from build123d import *

# Parameters (mm, degrees)
F0_R     = 25
F1_DEPTH = 43.4


with BuildPart() as f1:
    # F0 (on Front) → F1 (new body)
    with BuildSketch(Plane.XZ):
        Circle(F0_R)
        with BuildLine():
            ThreePointArc((-11.4564392374, 5), (0, 12.5), (11.4564392374, 5))
            Line((11.4564392374, 5), (15, 5))
            Line((15, 5), (15, -5))
            Line((15, -5), (11.4564392374, -5))
            ThreePointArc((11.4564392374, -5), (0, -12.5), (-11.4564392374, -5))
            Line((-11.4564392374, -5), (-15, -5))
            Line((-15, -5), (-15, 5))
            Line((-15, 5), (-11.4564392374, 5))
        make_face(mode=Mode.SUBTRACT)
        with BuildLine():
            ThreePointArc((-11.4564392374, -5), (-12.5, 0), (-11.4564392374, 5))
            Line((-11.4564392374, 5), (-15, 5))
            Line((-15, 5), (-15, -5))
            Line((-15, -5), (-11.4564392374, -5))
        make_face()
    extrude(amount=F1_DEPTH)


solid = f1.part
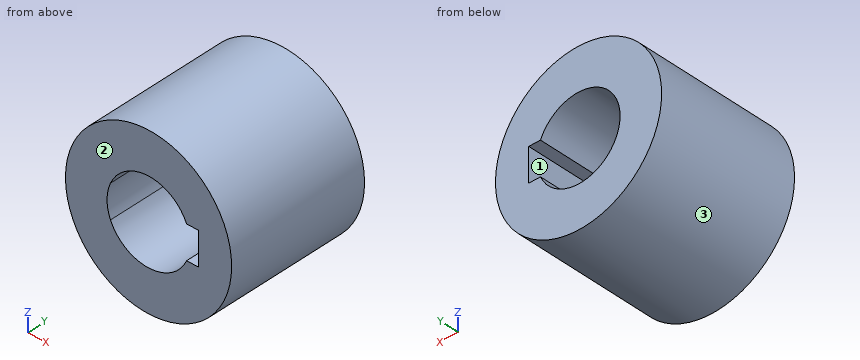
Read the model definition and answer for the solid it produces. Units are mm, in the model's axes. Face numbers are marked on the shaded views. Give positions to 0.01 mm unless a question says otherwise; leave off trailing zeros. Write each loop counter-clockwise with the first axis right and the second up, starting at its lowest first coordinate (ties: lowest second). Pieces come first, ordered by that corner, then holes. Notation, with made-up numbers: M -37.75,34 L -17.75,34 A20 cw -17.75,39 Z; hole C 58.25,23 d7. An arc over 180 degrees is marked long. One line per item, written item: value. Start each with the question number.
(1) Find section A-A (z = 0). Determine the outline of the cut face in (x, y).
(2) Find the intervals of material crossed by line 1 (Z direction, x = -0.5, y = -26) (3 decimals); line 2 (Z direction, x = 3, y = -40); line 3 (X direction, y = -38.5, z = -8), in increasing order.
(3) Find section C-C (y = -29.5). Determine the outline of the cut face in (x, z), plus the area to 3 significant figures.
(4) Determine the mould class of the marked faces 1, 2 and 3 for opening direction Z: pulls with the +Z half, pulls with the -Z half, needs draft (parallel to the pull), parting line crosses it, or undercut.
(5) Flat-ended cylindrical pins translate along their axes: pin 1 Ø4 at (x, y) = (12.5, -30) entering from +Z; pin 2 Ø12 at (x, y) = (0, -29.5) entering from +Z; pin 3 Ø1.5 at (y, z) = (-17, 12.5) entering from +X. Find the tip coordinate at first contact, or state that the pin passes through.
(6) Find section D-D (z = 20). Determine the outline of the cut face in (x, y).
(7) Find section B-B (x = 0). Determine the outline of the cut face in (y, z), plus the area to 4 significant figures.
Results below:
1. outline: M -25,-43.4 L -12.5,-43.4 L -12.5,0 L -25,0 Z; M 15,-43.4 L 25,-43.4 L 25,0 L 15,0 Z
2. line 1: z = -24.995 to -12.49, 12.49 to 24.995
2. line 2: z = -24.82 to -12.13, 12.13 to 24.82
2. line 3: x = -23.69 to -9.6, 9.6 to 23.69
3. outline: C 0,0 d50; hole M 11.46,-5 L 15,-5 L 15,5 L 11.46,5 A12.5 ccw long Z
3. area: 1,440 mm^2
4. face 1: undercut
4. face 2: needs draft
4. face 3: parting line crosses it
5. pin 1: stops at z = 22.69
5. pin 2: stops at z = 25
5. pin 3: stops at x = 22.07
6. outline: M -15,-43.4 L 15,-43.4 L 15,0 L -15,0 Z
7. outline: M -43.4,-25 L 0,-25 L 0,-12.5 L -43.4,-12.5 Z; M -43.4,12.5 L 0,12.5 L 0,25 L -43.4,25 Z
7. area: 1,085 mm^2
